Read the model definition and answer for the solid it produces. Units are mm, in the model's axes. A direction names the side the tool comes from. Coordinates: 2 decimals unless noted, no trailing zeros. Write each loop counter-clockwise with the first axis right and the second up, starting at its lowest first coordinate (ties: lowest second). Pieces come first, ordered by that corner, then holes.
Item 1: Straight lines are drawn through the part: probe 1 along X at (y, z) = (17, 11.75); probe 2 along Y at (x, z) = (88.35, -13.65); probe 3 along Z at (x, y) = (-95.5, 2.5). For each, find the intervals that lie inside material, in ascending order.
Item 2: Determine the mould class of faces 1 (the face through (90.45, 6.66, 14.09)), 2 (the face through (-134.5, 20.7, 0.1)), 3 (the face through (-124, 11, -12.85)), 4 (the face through (-15, 3, -9)) for opening direction Y: released by +Y, released by -Y, zero draft, split by the parting line, or undercut.
Item 3: Section D-D (y = 16.75) is taken. Give the vertices of the cut face in (x, z).
Item 4: Section B-B (x = -62.5) is taken. Give the vertices of the cut face in (y, z), then the cut area to 3 significant figures.
Item 5: Each of these flat-tipped pins is pushed along its axis until it touches: P1, Ø0.9, axis at x = -122.5, y = 21, coming from the -Z side; P2, Ø1, axis at x = -65, z = 8, coming from the +Y side; P3, Ø5, axis at x = 43, z = -1.5, coming from the -Y side; P4, Ø2.5, axis at y = 6, z = 10.5, coming from the +X side. Where does it stop, or does it pass through?
Item 6: A tool of negligible diameter and unlimited length cuts with its end or side. For faces 5 (the face through (-124, 2.15, -6)), 6 (the face through (101, 12, 0)), 7 (the face through (-1, 12, 12)), from which of +Z, -Z, +X, -X, +Y, -Y can it reach the whole face along a straight path? Write none if from no direction.
Item 7: Section A-A (z = 0) is taken. Give the vertices of the cut face in (x, y).
Item 8: Section C-C (y = 6) is taken. Give the vertices of the cut face in (x, z), then the cut area to 3 significant figures.
from build123d import *

# Parameters (mm, degrees)
SKETCH1_W           = 207
SKETCH1_H           = 30
BOSS_EXTRUDE1_DEPTH = 22
SHELL1_T            = -3
SKETCH2_W           = 207
SKETCH2_H           = 10
CUT_EXTRUDE1_DEPTH  = 3
SKETCH3_W           = 29.2
SKETCH3_H           = 21.2
BOSS_EXTRUDE2_DEPTH = 40
SKETCH4_W           = 25.7
SKETCH4_H           = 17.7
CUT_EXTRUDE2_DEPTH  = 40
CUT_EXTRUDE3_DEPTH  = 146.889718623
SKETCH6_W           = 30.3
SKETCH6_H           = 26.3
CUT_EXTRUDE4_DEPTH  = 12
SKETCH7_R           = 2.2
CUT_EXTRUDE5_DEPTH  = 149.243886889


with BuildPart() as part:
    # Sketch1 → Boss-Extrude1 (new body)
    with BuildSketch(Plane(origin=(0, 0, 0), x_dir=(1, 0, 0), z_dir=(0, 1, 0))):
        Rectangle(SKETCH1_W, SKETCH1_H)
    extrude(amount=BOSS_EXTRUDE1_DEPTH)

    # Shell1
    shell1_openings = [part.faces().sort_by_distance(p)[0] for p in [
        (0, 22, 0),
    ]]
    offset(amount=SHELL1_T, openings=shell1_openings, kind=Kind.INTERSECTION)

    # Sketch2 → Cut-Extrude1 (cut)
    with BuildSketch(Plane(origin=(0, 0, 0), x_dir=(-1, 0, 0), z_dir=(0, -1, 0))):
        Rectangle(SKETCH2_W, SKETCH2_H)
    extrude(amount=-CUT_EXTRUDE1_DEPTH, mode=Mode.SUBTRACT)

    # Sketch3 → Boss-Extrude2 (add)
    with BuildSketch(Plane.ZY.offset(103.5)):
        with Locations((0, 11)):
            Rectangle(SKETCH3_W, SKETCH3_H)
    extrude(amount=BOSS_EXTRUDE2_DEPTH)

    # Sketch4 → Cut-Extrude2 (cut)
    with BuildSketch(Plane.ZY.offset(143.5)):
        with Locations((0, 11)):
            Rectangle(SKETCH4_W, SKETCH4_H)
    extrude(amount=-CUT_EXTRUDE2_DEPTH, mode=Mode.SUBTRACT)

    # Sketch5 → Cut-Extrude3 (cut, through all)
    with BuildSketch(Plane(origin=(0, 21.6, 0), x_dir=(1, 0, 0), z_dir=(0, 1, 0))):
        with BuildLine():
            Line((-130.5, 4), (-116.5, 4))
            ThreePointArc((-116.5, 4), (-112.5, 0), (-116.5, -4))
            Line((-116.5, -4), (-130.5, -4))
            ThreePointArc((-130.5, -4), (-134.5, 0), (-130.5, 4))
        make_face()
    extrude(amount=-CUT_EXTRUDE3_DEPTH, mode=Mode.SUBTRACT)

    # Sketch6 → Cut-Extrude4 (cut)
    with BuildSketch(Plane(origin=(0, 0, 0), x_dir=(-1, 0, 0), z_dir=(0, -1, 0))):
        with Locations((-88.35, 0)):
            Rectangle(SKETCH6_W, SKETCH6_H)
    extrude(amount=-CUT_EXTRUDE4_DEPTH, mode=Mode.SUBTRACT)

    # Sketch7 → Cut-Extrude5 (cut, through all)
    with BuildSketch(Plane.XY.offset(15)):
        with Locations((88.35, 6)):
            Circle(SKETCH7_R)
    extrude(amount=-CUT_EXTRUDE5_DEPTH, mode=Mode.SUBTRACT)


solid = part.part
Established:
1. probe 1: x = -103.5 to -100.5, 100.5 to 103.5
1. probe 2: y = 0 to 3.8, 8.2 to 22
1. probe 3: z = -15 to -5, 5 to 15
2. face 1: undercut
2. face 2: zero draft
2. face 3: undercut
2. face 4: released by +Y
3. outline: (-143.5, -14.6) - (-103.5, -14.6) - (-103.5, -15) - (103.5, -15) - (103.5, 15) - (-103.5, 15) - (-103.5, 14.6) - (-143.5, 14.6) - (-143.5, 12.85) - (-103.5, 12.85) - (-103.5, -12.85) - (-143.5, -12.85) - close; hole (-100.5, -12) - (100.5, -12) - (100.5, 12) - (-100.5, 12) - close
4. outline: (0, -15) - (22, -15) - (22, -12) - (3, -12) - (3, -5) - (0, -5) - close; (0, 5) - (3, 5) - (3, 12) - (22, 12) - (22, 15) - (0, 15) - close
4. area: 174 mm2
5. P1: stops at z = -14.6
5. P2: stops at y = 3
5. P3: passes through
5. P4: stops at x = -100.5
6. face 5: -X
6. face 6: +X, -Y
6. face 7: +Y
7. outline: (-143.5, 0.4) - (-134.5, 0.4) - (-134.5, 2.15) - (-143.5, 2.15) - close; (-143.5, 19.85) - (-134.5, 19.85) - (-134.5, 21.6) - (-143.5, 21.6) - close; (-112.5, 0.4) - (-103.5, 0.4) - (-103.5, 2.15) - (-112.5, 2.15) - close; (-112.5, 19.85) - (-103.5, 19.85) - (-103.5, 3) - (-100.5, 3) - (-100.5, 22) - (-103.5, 22) - (-103.5, 21.6) - (-112.5, 21.6) - close; (100.5, 12) - (103.5, 12) - (103.5, 22) - (100.5, 22) - close
8. outline: (-143.5, -14.6) - (-103.5, -14.6) - (-103.5, -15) - (86.15, -15) - (86.15, -13.15) - (73.2, -13.15) - (73.2, -12) - (-100.5, -12) - (-100.5, 12) - (73.2, 12) - (73.2, 13.15) - (86.15, 13.15) - (86.15, 15) - (-103.5, 15) - (-103.5, 14.6) - (-143.5, 14.6) - (-143.5, 12.85) - (-103.5, 12.85) - (-103.5, -12.85) - (-143.5, -12.85) - close; (90.55, -15) - (103.5, -15) - (103.5, -13.15) - (90.55, -13.15) - close; (90.55, 13.15) - (103.5, 13.15) - (103.5, 15) - (90.55, 15) - close
8. area: 1,370 mm2
